Check sheet for the modelled part. Datum: model origin and axes. Units: mm. A direction names the side the tool comes from. Give positions to 0.01 mm unless a question says otherwise; leave off trailing zeros. Loops run counter-clockwise (first coordinate to the right, second up) from the corner with the lowest first, then second, coordinate; pieces in that order, holes last. Notation, with made-up numbers: (68, 61) - (120, 61) arc R16 ccw to (120, 89) - close; hole circle Ø10 at (-6.75, 45). An arc over 180 degrees is marked (long way). Answer in a Markdown table with one row per item. Add a question column.
(1) Sectioned sample at A-A on y = -42. Enter the section's corners in (x, z), then the cut area to 3 significant figures.
(2) Go/stop test with flat-tipped pins: P1, Ø5.5, axis at x = -1.5, z = -95, coming from the +Y side; P2, Ø2, axis at y = -2.5, z = 34.5, coming from the +X side; P3, Ø2, axis at x = 9, y = -20, coming from the -Z side; P4, Ø1.2, axis at y = -1, z = -95.5, coming from the +X side. Record where each tip stops, or that it passes through.
(3) Sectioned sample at B-B on x = 0. State how many separate pieces and enclosed holes the cut face has, then the cut area to 3 significant figures.
(4) Draft check along X on faces 3 (the face through (6.83, -14.26, 2.15)), 4 (the face through (0, -8, 49)), 5 (the face through (0, -4, 96)). Enter one of: released by +X, released by -X, zero draft, split by the parting line, or undercut.
(5) Set-up check for faces 1 (the face through (-4, -2, -1)), 2 (the face through (4.77, -4.83, -88.5)): record each of +Z, -Z, +X, -X, +Y, -Y from which the full face is reachable in a straight line by a thin tool's end or side.
(6) Sectioned sample at D-D on y = -19. Enter the section's corners in (x, z), then the cut area to 3 significant figures.
(7) Thickness scan on L1, parallel to Y at x = -7.5, z = 41.5; L2, parallel to X at y = -4, z = 90; L3, parallel to Y at x = 1.75, z = 40.5. Record the ranges inside material, lowest first.
from build123d import *

# Parameters (mm, degrees)
F0_W      = 16
F0_H      = 196
F1_DEPTH  = 8
F1_TAPER  = -3
F2_W      = 8
F2_H      = 200
F3_DEPTH  = 4
F4_R      = 5
F5_DEPTH  = 25.4
F6_R      = 8.4192622343
F8_R      = 4.0010936275
F15_R     = 17.8032930924
F16_DEPTH = 25
F14_R     = 17.9120379097
F17_DEPTH = 25


with BuildPart() as f1:
    # F0 (on Front) → F1 (new body)
    with BuildSketch(Plane.XZ):
        Rectangle(F0_W, F0_H)
    extrude(amount=F1_DEPTH, taper=F1_TAPER)

    # F2 (on face) → F3 (cut)
    with BuildSketch(Plane.XZ):
        Rectangle(F2_W, F2_H)
    extrude(amount=F3_DEPTH, mode=Mode.SUBTRACT)

    # F4 (on Front) → F5 (cut)
    with BuildSketch(Plane.XZ):
        with Locations((0, 90)):
            Circle(F4_R)
        with Locations((0, -90)):
            Circle(F4_R)
    extrude(amount=F5_DEPTH, mode=Mode.SUBTRACT)

    # F6 (on face) → F9 section 0
    with BuildSketch(Plane.XZ.offset(8)):
        Circle(F6_R)
    # F8 (on offset) → F9 section 1
    with BuildSketch(Plane.XZ.offset(30)):
        Circle(F8_R)
    loft()

    # F10 (on Top) → F11 (revolve)
    with BuildSketch(Plane.XY):
        with BuildLine():
            Line((0, -45), (0, -15))
            ThreePointArc((0, -15), (-15, -30), (0, -45))
        make_face()
    revolve(axis=Axis((0, -30, 0), (0, -1, 0)))

    # F15 (on offset) → F16 (cut)
    with BuildSketch(Plane.YZ.offset(25)):
        with Locations((-29.9964938313, 0)):
            Circle(F15_R)
    extrude(amount=F16_DEPTH, mode=Mode.SUBTRACT)

    # F14 (on offset) → F17 (cut)
    with BuildSketch(Plane.YZ.offset(-25)):
        with Locations((-29.9462787807, 0)):
            Circle(F14_R)
    extrude(amount=-F17_DEPTH, mode=Mode.SUBTRACT)


solid = f1.part
Reply:
| question | item | result |
|---|---|---|
| 1 | outline | circle Ø18 at (0, 0) |
| 1 | area | 254 mm^2 |
| 2 | P1 | y = 0 |
| 2 | P2 | x = 8.18 |
| 2 | P3 | z = -8.36 |
| 2 | P4 | x = 8.08 |
| 3 | separate pieces | 3 |
| 3 | enclosed holes | 0 |
| 3 | area | 1,530 mm^2 |
| 4 | face 3 | split by the parting line |
| 4 | face 4 | zero draft |
| 4 | face 5 | undercut |
| 5 | face 1 | +Z, -Z, +Y |
| 5 | face 2 | +Y, -Y |
| 6 | outline | circle Ø20.4 at (0, 0) |
| 6 | area | 327 mm^2 |
| 7 | L1 | -8 to 0 |
| 7 | L2 | -8.21 to -5, 5 to 8.21 |
| 7 | L3 | -8 to -4 |
